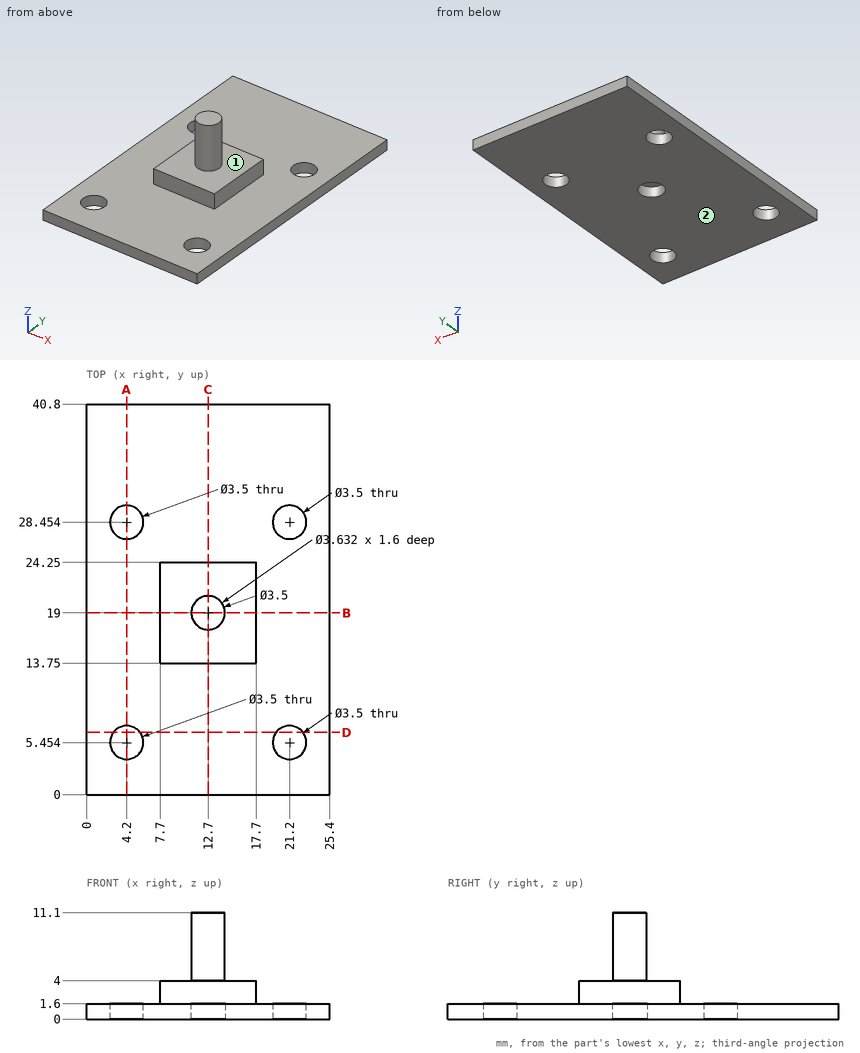
Here's the drawing with two shaded views (mm, measured from the low corner). I have some questions. A direction names the side the tool comes from. Round coordinates to 2 decimals unless told otherwise and drop trailing zeros. Write each loop counter-clockwise with the first axis right and the second up, starting at its lowest first coordinate (ties: lowest second). Pieces come first, ordered by that corner, then holes. Notation, with made-up numbers: M -0.5,33.5 L 26.5,33.5 A36 ccw 26.5,71.5 Z; hole C -27,-7.5 d6. An arc over 180 degrees is marked long. Use CSV: the item, a comma, the result in double quotes.
(1) Imagine slicing it at D-D (y = 6.5). Write out the boundary of the cut face in (x, z).
Check values:
outline,"M 0,0 L 2.8,0 L 2.8,1.6 L 0,1.6 Z; M 5.6,0 L 19.8,0 L 19.8,1.6 L 5.6,1.6 Z; M 22.6,0 L 25.4,0 L 25.4,1.6 L 22.6,1.6 Z"
(2) On a 3-axis mill with a long thin cutter (end or side, diameter ignored), from which of +Z, -Z, +X, -X, +Y, -Y can I reach the whole of each face in a straight line? I mean the marked faces 1 and 2. Say none if no direction works.
Check values:
face 1,"+Z"
face 2,"-Z, +X, -X, +Y, -Y"
(3) I need wall thicknesses on line 1 along Y through (x, z) = (12.7, 1); line 2 along Y through (x, z) = (4.2, 0.55) (1 decimal); line 3 along Y through (x, z) = (11.5, 2.25). Which ranges of each line are inside material? Lowest first, please.
Check values:
line 1,"0 to 17.18, 20.82 to 40.8"
line 2,"0 to 3.7, 7.2 to 26.7, 30.2 to 40.8"
line 3,"13.75 to 24.25"
(4) I'm going to push flat-ended pins straight in: pin 1 (5 mm diameter, centred on x = 11.5, y = 4.5, fed in from +Z); pin 2 (3 mm diameter, centred on x = 6.5, y = 14, fed in from +Z); pin 3 (1.2 mm diameter, centred on x = 11, z = 2.5, fed in from -Y); pin 4 (3 mm diameter, centred on x = 4.2, y = 5.45, fed in from +Z) (3 decimals). Where does each tip first touch, or does it pass through?
Check values:
pin 1,"z = 1.6"
pin 2,"z = 4"
pin 3,"y = 13.75"
pin 4,"through"
(5) Imagine slicing it at A-A (x = 4.2). Write out the boundary of the cut face in (y, z) (1 decimal).
Check values:
outline,"M 0,0 L 3.7,0 L 3.7,1.6 L 0,1.6 Z; M 7.2,0 L 26.7,0 L 26.7,1.6 L 7.2,1.6 Z; M 30.2,0 L 40.8,0 L 40.8,1.6 L 30.2,1.6 Z"
(6) Imagine slicing it at B-B (y = 19). Write out the boundary of the cut face in (x, z).
Check values:
outline,"M 0,0 L 10.88,0 L 10.88,1.6 L 14.52,1.6 L 14.52,0 L 25.4,0 L 25.4,1.6 L 17.7,1.6 L 17.7,4 L 14.45,4 L 14.45,11.1 L 10.95,11.1 L 10.95,4 L 7.7,4 L 7.7,1.6 L 0,1.6 Z"
(7) Imagine slicing it at C-C (x = 12.7). Write out the boundary of the cut face in (y, z).
Check values:
outline,"M 0,0 L 17.18,0 L 17.18,1.6 L 20.82,1.6 L 20.82,0 L 40.8,0 L 40.8,1.6 L 24.25,1.6 L 24.25,4 L 20.75,4 L 20.75,11.1 L 17.25,11.1 L 17.25,4 L 13.75,4 L 13.75,1.6 L 0,1.6 Z"
